from build123d import *

# Parameters (mm, degrees)
SKETCH_R      = 25
PAD_DEPTH     = 2
SKETCH002_R   = 25
SKETCH002_R_2 = 6
PAD001_DEPTH  = 58


with BuildPart() as part:
    # Sketch → Pad (new body)
    with BuildSketch(Plane.XY):
        Circle(SKETCH_R)
    extrude(amount=PAD_DEPTH)

    # Sketch002 (on Face3 of Pad) → Pad001 (join)
    with BuildSketch(Plane.XY.offset(2)):
        Circle(SKETCH002_R)
        with Locations((0, 17)):
            Circle(SKETCH002_R_2, mode=Mode.SUBTRACT)
        with Locations((-12.758063, 11.235294)):
            Circle(SKETCH002_R_2, mode=Mode.SUBTRACT)
        with Locations((12.758063, 11.235294)):
            Circle(SKETCH002_R_2, mode=Mode.SUBTRACT)
        with BuildLine():
            ThreePointArc((-23, 0), (0, -23), (23, 0))
            ThreePointArc((23, 0), (22.052404, 2.287698), (19.764706, 3.235294))
            Line((19.764706, 3.235294), (12.758063, 3.235294))
            ThreePointArc((6.754269, 5.948097), (9.463945, 3.944973), (12.758063, 3.235294))
            ThreePointArc((6.754269, 5.948097), (3.705882, 8.201612), (0, 9))
            ThreePointArc((0, 9), (-3.705882, 8.201612), (-6.754269, 5.948097))
            ThreePointArc((-12.758063, 3.235294), (-9.463945, 3.944973), (-6.754269, 5.948097))
            Line((-19.764706, 3.235294), (-12.758063, 3.235294))
            ThreePointArc((-19.764706, 3.235294), (-22.052404, 2.287698), (-23, 0))
        make_face(mode=Mode.SUBTRACT)
    extrude(amount=PAD001_DEPTH)


solid = part.part
Model file for the job. Use its own axes, mm. A direction names the side the tool comes from. Coordinates: 2 decimals unless noted, no trailing zeros. Order: outer loops, then holes, each group sorted by start corner. A loop starts at its lowest first (then second) coordinate and runs counter-clockwise, first axis right, second up. Notation, with made-up numbers: M 62.25,27 L 70.25,27 A22 ccw 70.25,63 Z; hole C 70,86.25 d6. An arc over 180 degrees is marked long. Return JSON: item names as keys, results as strings.
1. Flat gauge pins, fed straight in: pin 1 (7.5 mm diameter, centred on x = 17, z = 35.5, fed in from -Y); pin 2 (5 mm diameter, centred on x = 5, z = 33, fed in from -Y); pin 3 (3 mm diameter, centred on y = -13.5, z = 41.5, fed in from +X). Where does each tip first touch, or does it go through?
Ans:
{"pin 1": "y = -21.2", "pin 2": "y = -24.87", "pin 3": "x = 21.93"}
2. Saw through at A-A (z = 39). Give the cut face in (x, y).
Ans:
{"outline": "C 0,0 d50; hole M -23,0 A23 ccw 23,0 A3.24 ccw 19.76,3.24 L 12.76,3.24 A8 cw 6.75,5.95 A9 ccw -6.75,5.95 A8 cw -12.76,3.24 L -19.76,3.24 A3.24 ccw Z; hole C -12.76,11.24 d12; hole C 0,17 d12; hole C 12.76,11.24 d12"}
3. Saw through at C-C (y = -13.5). Give the cut face in (x, z).
Ans:
{"outline": "M -21.04,0 L 21.04,0 L 21.04,60 L 18.62,60 L 18.62,2 L -18.62,2 L -18.62,60 L -21.04,60 Z"}
4. Pull direction Y, two halves, no side cores. Call faces 3 (the face through (0, 0, 0)), 4 (the face through (23.846, 7.509, 29.58)), 5 (the face through (13, 11, 2)): +Y half, -Y half, draft (parallel to the pull), parting line (faces both ways), or undercut.
Ans:
{"face 3": "draft", "face 4": "parting line", "face 5": "undercut"}
5. Saw through at B-B (x = 15.5). Give the cut face in (y, z).
Ans:
{"outline": "M -19.62,0 L 19.62,0 L 19.62,60 L 16.57,60 L 16.57,2 L 5.9,2 L 5.9,60 L 3.24,60 L 3.24,2 L -16.99,2 L -16.99,60 L -19.62,60 Z"}
6. Saw through at D-D (y = 13.5). Give the cut face in (x, z), and give its area (3 significant figures).
Ans:
{"outline": "M -21.04,0 L 21.04,0 L 21.04,60 L 18.31,60 L 18.31,2 L 7.2,2 L 7.2,60 L 4.87,60 L 4.87,2 L -4.87,2 L -4.87,60 L -7.2,60 L -7.2,2 L -18.31,2 L -18.31,60 L -21.04,60 Z", "area": "671 mm^2"}
7. Tool access for faces 1 (the face through (-0.1, 9.4, 60)), 2 (the face through (-9.507, 3.926, 30.594)): list every direction of +Z, -Z, +X, -X, +Y, -Y with a clear straight run to the whole face (end or side of a thin tool).
Ans:
{"face 1": "+Z, +X, -X, +Y, -Y", "face 2": "+Z"}
8. Drill centre lines: probe 1 along Y at (x, z) = (-11.5, 11); probe 2 along Y at (x, z) = (10, 54); probe 3 along X at (y, z) = (7, 47). Where is each one in solid material? Low to high.
Ans:
{"probe 1": "-22.2 to -19.92, 3.33 to 5.37, 17.1 to 22.2", "probe 2": "-22.91 to -20.71, 3.73 to 5.91, 16.56 to 22.91", "probe 3": "-24 to -17.01, -8.51 to -5.66, 5.66 to 8.51, 17.01 to 24"}
